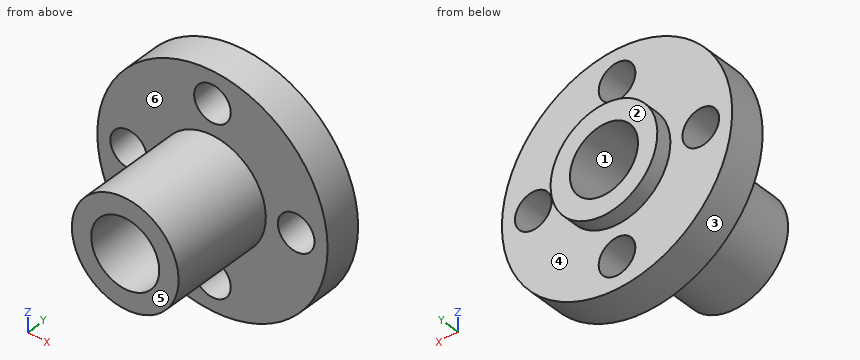
```python
from build123d import *

# Parameters (mm, degrees)
SKETCH1_R                = 11
BOSS_EXTRUDE1_DEPTH      = 3.5
BOSS_EXTRUDE2_DEPTH      = 1.5
BOSS_EXTRUDE2_DEPTH_BACK = 13.5
SKETCH2_R                = 5.1
SKETCH3_R                = 3.25
CUT_EXTRUDE1_DEPTH       = 22.610182785
SKETCH4_R                = 1.75
CUT_EXTRUDE2_DEPTH       = 21.597329924


with BuildPart() as part:
    # Sketch1 → Boss-Extrude1 (new body)
    with BuildSketch(Plane(origin=(0, 0, 0), x_dir=(1, 0, 0), z_dir=(0, 1, 0))):
        with Locations(Location((0, 0, 0), (0, 0, 270))):
            Circle(SKETCH1_R)
    extrude(amount=BOSS_EXTRUDE1_DEPTH)

    # Sketch2 → Boss-Extrude2 (add, two sides: drawn at the far end of the back side and taken through both)
    with BuildSketch(Plane(origin=(0, 3.5, 0), x_dir=(1, 0, 0), z_dir=(0, 1, 0)).offset(-BOSS_EXTRUDE2_DEPTH_BACK)):
        with Locations(Location((0, 0, 0), (0, 0, 270))):
            Circle(SKETCH2_R)
    extrude(amount=BOSS_EXTRUDE2_DEPTH + BOSS_EXTRUDE2_DEPTH_BACK)

    # Sketch3 → Cut-Extrude1 (cut, through all)
    with BuildSketch(Plane(origin=(0, 5, 0), x_dir=(1, 0, 0), z_dir=(0, 1, 0))):
        with Locations(Location((0, 0, 0), (0, 0, 270))):
            Circle(SKETCH3_R)
    extrude(amount=-CUT_EXTRUDE1_DEPTH, mode=Mode.SUBTRACT)

    # Sketch4 → Cut-Extrude2 (cut, through all)
    with BuildSketch(Plane(origin=(0, 3.5, 0), x_dir=(1, 0, 0), z_dir=(0, 1, 0))):
        with Locations(Location((-8, 0, 0), (0, 0, 270))):
            Circle(SKETCH4_R)
        with Locations(Location((0, 8, 0), (0, 0, 270))):
            Circle(SKETCH4_R)
        with Locations(Location((8, 0, 0), (0, 0, 270))):
            Circle(SKETCH4_R)
        with Locations(Location((0, -8, 0), (0, 0, 270))):
            Circle(SKETCH4_R)
    extrude(amount=-CUT_EXTRUDE2_DEPTH, mode=Mode.SUBTRACT)


solid = part.part
```
Can you work these out from the model? Positions are in its coordinate system, mm. Face numbers are marked on the shaded views. A direction names the side the tool comes from. Coordinates: 2 decimals unless noted, no trailing zeros. Write each loop counter-clockwise with the first axis right and the second up, starting at its lowest first coordinate (ties: lowest second). Pieces come first, ordered by that corner, then holes. Notation, with made-up numbers: (66, 4) - (109, 4) arc R18 ccw to (109, 35) - close; hole circle Ø5 at (-23, -28.75). An arc over 180 degrees is marked (long way). Return JSON: item names as keys, results as strings.
Q1. Please list where these lines run through material, in increasing order: L1, parallel to X at y = 2.6, z = 0; L2, parallel to Z at x = 1, y = 1.75; L3, parallel to X at y = 1.5, z = 0.75. Write a range as from..to.
Computed values:
{"L1": "x = -11..-9.75, -6.25..-3.25, 3.25..6.25, 9.75..11", "L2": "z = -10.95..-9.44, -6.56..-3.09, 3.09..6.56, 9.44..10.95", "L3": "x = -10.97..-9.58, -6.42..-3.16, 3.16..6.42, 9.58..10.97"}
Q2. If we section it at C-C (x = 8.5): Please give me the cut outline in (y, z), then the cut area to 3 significant figures.
Computed values:
{"outline": "(0, -6.98) - (3.5, -6.98) - (3.5, -1.68) - (0, -1.68) - close; (0, 1.68) - (3.5, 1.68) - (3.5, 6.98) - (0, 6.98) - close", "area": "37.1 mm2"}
Q3. Thinking about a two-plate mould opening in Z: for the marked faces 1, 2 and 3, which applies, +Z half, -Z half, draft (parallel to the pull), parting line (faces both ways), or undercut?
Computed values:
{"face 1": "undercut", "face 2": "draft", "face 3": "parting line"}
Q4. If we section it at D-D (z = -2.25): Please give me the cut outline in (x, y), then the cut area to 3 significant figures.
Computed values:
{"outline": "(-10.77, 0) - (-4.58, 0) - (-4.58, -10) - (-2.35, -10) - (-2.35, 5) - (-4.58, 5) - (-4.58, 3.5) - (-10.77, 3.5) - close; (2.35, -10) - (4.58, -10) - (4.58, 0) - (10.77, 0) - (10.77, 3.5) - (4.58, 3.5) - (4.58, 5) - (2.35, 5) - close", "area": "110 mm2"}
Q5. I'm going to push flat-ended pins straight in: pin 1 Ø4 at (x, z) = (-8, 0) entering from -Y; pin 2 Ø2 at (x, z) = (8, 0) entering from -Y; pin 3 Ø1 at (y, z) = (-1, -2) entering from +X; pin 4 Ø2 at (x, y) = (-7, 1.5) entering from +Z. Where does each tip first touch, or does it pass through?
Computed values:
{"pin 1": "stops at y = 0", "pin 2": "passes through", "pin 3": "stops at x = 4.87", "pin 4": "stops at z = 9.22"}
Q6. On a 3-axis mill with a long thin cutter (end or side, diameter ignored), from which of +Z, -Z, +X, -X, +Y, -Y can I reach the whole of each face in a straight line? I mean the marked faces 4, 5 and 6. Say none if no direction works.
Computed values:
{"face 4": "+Y", "face 5": "+Z, -Z, +X, -X, -Y", "face 6": "-Y"}
Q7. If we section it at A-A (z = 0): Please give me the cut outline in (x, y), then the cut area to 3 significant figures.
Computed values:
{"outline": "(-11, 0) - (-9.75, 0) - (-9.75, 3.5) - (-11, 3.5) - close; (-6.25, 0) - (-5.1, 0) - (-5.1, -10) - (-3.25, -10) - (-3.25, 5) - (-5.1, 5) - (-5.1, 3.5) - (-6.25, 3.5) - close; (3.25, -10) - (5.1, -10) - (5.1, 0) - (6.25, 0) - (6.25, 3.5) - (5.1, 3.5) - (5.1, 5) - (3.25, 5) - close; (9.75, 0) - (11, 0) - (11, 3.5) - (9.75, 3.5) - close", "area": "72.3 mm2"}
Q8. If we section it at B-B (x = 0): Please give me the cut outline in (y, z).
Computed values:
{"outline": "(-10, -5.1) - (0, -5.1) - (0, -6.25) - (3.5, -6.25) - (3.5, -5.1) - (5, -5.1) - (5, -3.25) - (-10, -3.25) - close; (-10, 3.25) - (5, 3.25) - (5, 5.1) - (3.5, 5.1) - (3.5, 6.25) - (0, 6.25) - (0, 5.1) - (-10, 5.1) - close; (0, -11) - (3.5, -11) - (3.5, -9.75) - (0, -9.75) - close; (0, 9.75) - (3.5, 9.75) - (3.5, 11) - (0, 11) - close"}
